Here's the drawing with two shaded views (mm, measured from the low corner). I have some questions. A direction names the side the tool comes from. Give positions to 0.01 mm unless a question says otherwise; leave off trailing zeros. Loops run counter-clockwise (first coordinate to the right, second up) from the corner with the lowest first, then second, coordinate; pieces in that order, holes last. Notation, with made-up numbers: M 3,22 L 57,22 A10 ccw 57,30 Z; hole C 25.5,28 d4. An arc over 180 degrees is marked long. Write item = value, one per line. Start each with the question number.
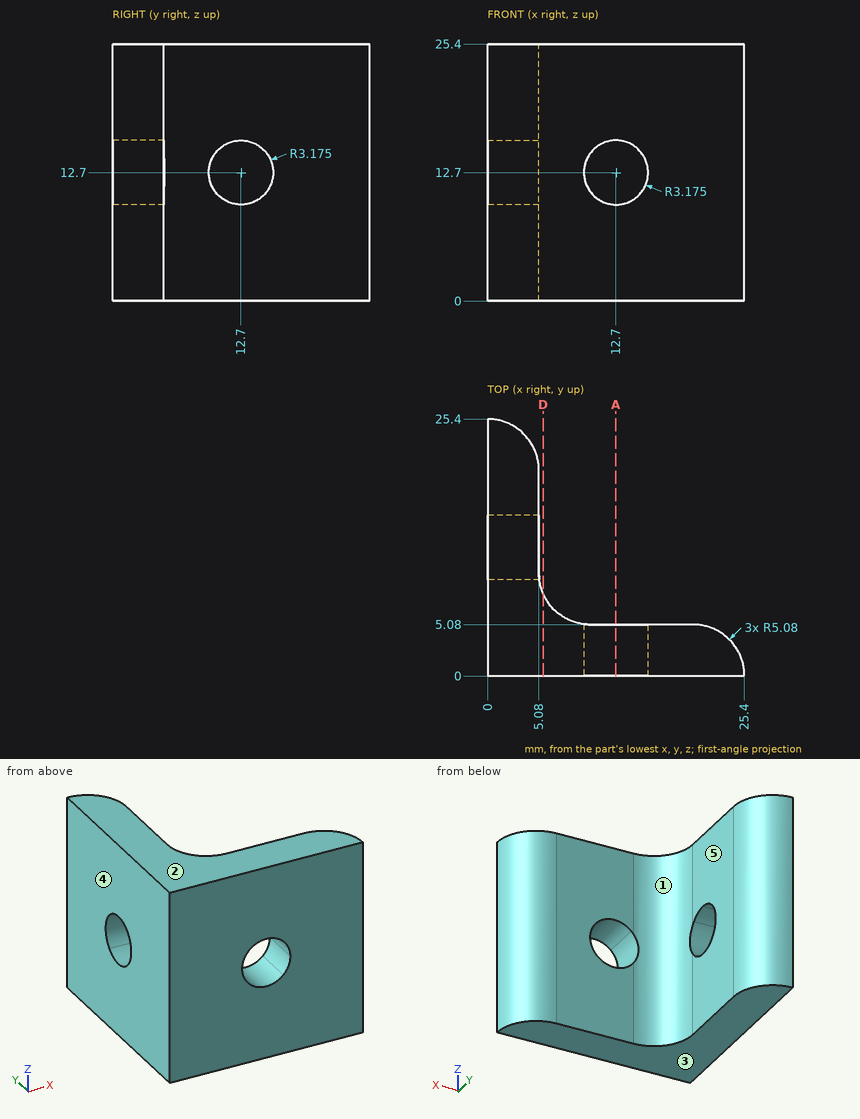
Q1. On a 3-axis mill with a long thin cutter (end or side, diameter ignored), from which of +Z, -Z, +X, -X, +Y, -Y can I reach the whole of each face in a straight line? I mean the marked faces 4 and 5. Say none if no direction works.
Q2. If I drill on line 1 along X through (y, z) = (14.75, 7); line 2 along Z through (x, y) = (3, 15), over which ranges is the centre line in solid material (lowest first)?
Q3. Will these pins go through, and if not, where does the flat tip stop? pin 1 (1.5 mm diameter, centred on x = 21.5, z = 16, fed in from +Y); pin 2 (5 mm diameter, centred on y = 10, z = 12, fed in from +X); pin 3 (3 mm diameter, centred on x = 13.5, z = 11.5, fed in from +Y); pin 4 (1.5 mm diameter, centred on y = 22.5, z = 11.5, fed in from +X).
Q4. We'd pull the mould along Z, two halves only. Please class the marked faces 1, 2 and 3: pulls with the +Z half, pulls with the -Z half, needs draft (parallel to the pull), parting line crosses it, or undercut.
Q5. If we section it at A-A, the plane x = 12.7: List the corners of the cut face in (y, z) for me (3 decimals), then the cut area to 3 significant figures.
Q6. If we section it at D-D, the plane x = 5.5: List the corners of the cut face in (y, z) for me, then the cut area to 3 significant figures.
Resolved:
q1.face_4 = +Z, -Z, -X, +Y, -Y
q1.face_5 = +Z, -Z, +X, +Y
q2.line_1 = 0 to 5.08
q2.line_2 = 0 to 10.51, 14.89 to 25.4
q3.pin_1 = 5.06
q3.pin_2 = 5.83
q3.pin_3 = through
q3.pin_4 = 4.87
q4.face_1 = needs draft
q4.face_2 = pulls with the +Z half
q4.face_3 = pulls with the -Z half
q5.outline = M 0,0 L 5.08,0 L 5.08,9.525 L 0,9.525 Z; M 0,15.875 L 5.08,15.875 L 5.08,25.4 L 0,25.4 Z
q5.area = 96.8 mm²
q6.outline = M 0,0 L 8.14,0 L 8.14,25.4 L 0,25.4 Z
q6.area = 207 mm²
